For this review, take the finished solid that the model builds, in its own axes (mm). A direction names the side the tool comes from. Round coordinates to 2 decimals unless told otherwise and drop trailing zeros. Loops run counter-clockwise (first coordinate to the right, second up) from the corner with the lowest first, then second, coordinate; pieces in that order, holes last. Notation, with made-up numbers: (-8, 78.25) -> (49, 78.25) arc R36 ccw to (49, 115.25) -> close; hole circle Ø10 at (-12.5, -39). An arc over 180 degrees is marked (long way). Write each question's results on one line, items separated by ' | '.
```python
from build123d import *

# Parameters (mm, degrees)
SKETCH1_R           = 2
BOSS_EXTRUDE1_DEPTH = 37.86
CUT_EXTRUDE1_DEPTH  = 28.86


with BuildPart() as part:
    # Sketch1 → Boss-Extrude1 (new body)
    with BuildSketch(Plane(origin=(0, 0, 0), x_dir=(1, 0, 0), z_dir=(0, 1, 0))):
        with BuildLine():
            Line((-12, 6), (12, 6))
            ThreePointArc((12, 6), (18, 0), (12, -6))
            Line((12, -6), (-12, -6))
            ThreePointArc((-12, -6), (-18, 0), (-12, 6))
        make_face()
        with Locations(Location((-12, 0, 0), (0, 0, 270))):
            Circle(SKETCH1_R, mode=Mode.SUBTRACT)
        with Locations(Location((12, 0, 0), (0, 0, 270))):
            Circle(SKETCH1_R, mode=Mode.SUBTRACT)
    extrude(amount=BOSS_EXTRUDE1_DEPTH)

    # Sketch2 → Cut-Extrude1 (cut)
    with BuildSketch(Plane.XZ):
        Polygon((-13.833087105, 3.175), (-15.666174209, 0), (-13.833087105, -3.175), (-10.166912895, -3.175), (-8.333825791, 0), (-10.166912895, 3.175), align=None)
    cut_extrude1 = extrude(amount=-CUT_EXTRUDE1_DEPTH, mode=Mode.SUBTRACT)

    # Mirror1: Cut-Extrude1 across plane
    add(cut_extrude1.mirror(Plane(origin=(0, 0, 0), x_dir=(0, 0, 1), z_dir=(1, 0, 0))), mode=Mode.SUBTRACT)


solid = part.part
```
1. Draft analysis for pull direction Z (two halves, no side actions). For faces 3 (the face through (-18, 19, 0)), 4 (the face through (12, 14, -3.175)), 5 (the face through (0, 19, 6)), state which applies: released by +Z, released by -Z, zero draft, split by the parting line, or undercut.
Values found:
face 3: split by the parting line | face 4: undercut | face 5: released by +Z
2. Tool access review of faces 1 (the face through (18, 19, 0)), 2 (the face through (-12, 14, -3.175)): name each direction out of +Z, -Z, +X, -X, +Y, -Y from which nothing blocks a thin tool from reaching the whole face with its end or side.
Values found:
face 1: +X, +Y, -Y | face 2: -Y
3. Consider section A-A (y = 19). State the section outline as (x, z) points (3 decimals), plus the area to 3 significant figures.
Values found:
outline: (-12, -6) -> (12, -6) arc R6 ccw to (12, 6) -> (-12, 6) arc R6 ccw to start; hole (-15.666, 0) -> (-13.833, -3.175) -> (-10.167, -3.175) -> (-8.334, 0) -> (-10.167, 3.175) -> (-13.833, 3.175) -> close; hole (8.334, 0) -> (10.167, -3.175) -> (13.833, -3.175) -> (15.666, 0) -> (13.833, 3.175) -> (10.167, 3.175) -> close | area: 331 mm2
4. For pin 1 (1.1 mm diameter, centred on x = -13, y = 12, fed in from -Z); pin 2 (1 mm diameter, centred on x = 11, z = 0, fed in from -Y); pin 3 (1.9 mm diameter, centred on x = 13, z = -1.5, fed in from -Y), all flat-tipped, find the tip position at first contact; note any pin that passes through.
Values found:
pin 1: stops at z = -5.98 | pin 2: passes through | pin 3: stops at y = 28.86
5. Consider section B-B (y = 35.5). State the section outline as (x, z) points, plus the area to 3 significant figures.
Values found:
outline: (-12, -6) -> (12, -6) arc R6 ccw to (12, 6) -> (-12, 6) arc R6 ccw to start; hole circle Ø4 at (-12, 0); hole circle Ø4 at (12, 0) | area: 376 mm2
6. Consider section C-C (z = -5). State the section outline as (x, y) points, plus the area to 3 significant figures.
Values found:
outline: (-15.32, 0) -> (15.32, 0) -> (15.32, 37.86) -> (-15.32, 37.86) -> close | area: 1,160 mm2
7. To check wall thickness, follow probe 1 along Z at (x, y) = (12, 34.75); probe 2 along X at (y, z) = (33, 0); probe 3 along X at (y, z) = (18, 2.75). State the ranges of each line that lie inside material, in increasing order.
Values found:
probe 1: z = -6 to -2, 2 to 6 | probe 2: x = -18 to -14, -10 to 10, 14 to 18 | probe 3: x = -17.33 to -14.08, -9.92 to 9.92, 14.08 to 17.33
